Geometry: final body of the model. Coordinates: model frame, mm. Coordinates: 2 decimals unless noted, no trailing zeros. Order: outer loops, then holes, each group sorted by start corner. A loop starts at its lowest first (then second) coordinate and runs counter-clockwise, first axis right, second up. Notation, with made-up numbers: M -8,30.25 L 42,30.25 A30 cw 42,58.25 Z; hole C 0,-5 d2. An arc over 180 degrees is marked long. Write item = value, one per line.
from build123d import *

# Parameters (mm, degrees)
SKETCH5_W           = 381
SKETCH5_H           = 195.58
BOSS_EXTRUDE2_DEPTH = 6.35
SKETCH6_W           = 209.55
SKETCH6_H           = 195.58
BOSS_EXTRUDE3_DEPTH = 6.35
SKETCH7_W           = 209.55
SKETCH7_H           = 195.58
BOSS_EXTRUDE4_DEPTH = 6.35
SKETCH9_W           = 146.05
SKETCH9_H           = 50.8
CUT_EXTRUDE1_DEPTH  = 7.35


with BuildPart() as part:
    # Sketch5 → Boss-Extrude2 (new body)
    with BuildSketch(Plane(origin=(0, 0, 0), x_dir=(1, 0, 0), z_dir=(0, 1, 0))):
        with Locations((190.5, 97.79)):
            Rectangle(SKETCH5_W, SKETCH5_H)
    extrude(amount=BOSS_EXTRUDE2_DEPTH)

    # Sketch6 → Boss-Extrude3 (add)
    with BuildSketch(Plane(origin=(0, 0, 0), x_dir=(1, 0, 0), z_dir=(0, 1, 0))):
        with Locations((485.775, 97.79)):
            Rectangle(SKETCH6_W, SKETCH6_H)
    extrude(amount=BOSS_EXTRUDE3_DEPTH)

    # Sketch7 → Boss-Extrude4 (add)
    with BuildSketch(Plane(origin=(0, 0, 0), x_dir=(1, 0, 0), z_dir=(0, 1, 0))):
        with Locations((-104.775, 97.79)):
            Rectangle(SKETCH7_W, SKETCH7_H)
    extrude(amount=BOSS_EXTRUDE4_DEPTH)

    # Sketch9 → Cut-Extrude1 (cut, through all)
    with BuildSketch(Plane(origin=(0, 6.35, 0), x_dir=(1, 0, 0), z_dir=(0, 1, 0))):
        with Locations((190.5, 170.18)):
            Rectangle(SKETCH9_W, SKETCH9_H)
    extrude(amount=-CUT_EXTRUDE1_DEPTH, mode=Mode.SUBTRACT)


solid = part.part
1) Pin query (flat end, axial travel): pin 1 (3 mm diameter, centred on x = 166, y = 4, fed in from -Z); pin 2 (1.5 mm diameter, centred on x = 166.5, y = 3.5, fed in from +Z). Return the tip coordinate at first contact, or that it passes through.
Numbers:
pin_1 = -144.78
pin_2 = 0
2) Section B-B, the plane x = 220. Return loops of the section in (y, z).
Numbers:
outline = M 0,-144.78 L 6.35,-144.78 L 6.35,0 L 0,0 Z
3) Section A-A, the plane y = 2.25. Return loops of the section in (x, z) (3 decimals), and give its area (3 significant figures).
Numbers:
outline = M -209.55,-195.58 L 117.475,-195.58 L 117.475,-144.78 L 263.525,-144.78 L 263.525,-195.58 L 590.55,-195.58 L 590.55,0 L -209.55,0 Z
area = 149,000 mm²
4) Line query: L1, parallel to X at y = 2.75, z = -152 (3 decimals); L2, parallel to Z at x = 255.5, y = 3.5. Output: solid intervals per line, ascending.
Numbers:
L1 = -209.55 to 117.475, 263.525 to 590.55
L2 = -144.78 to 0
